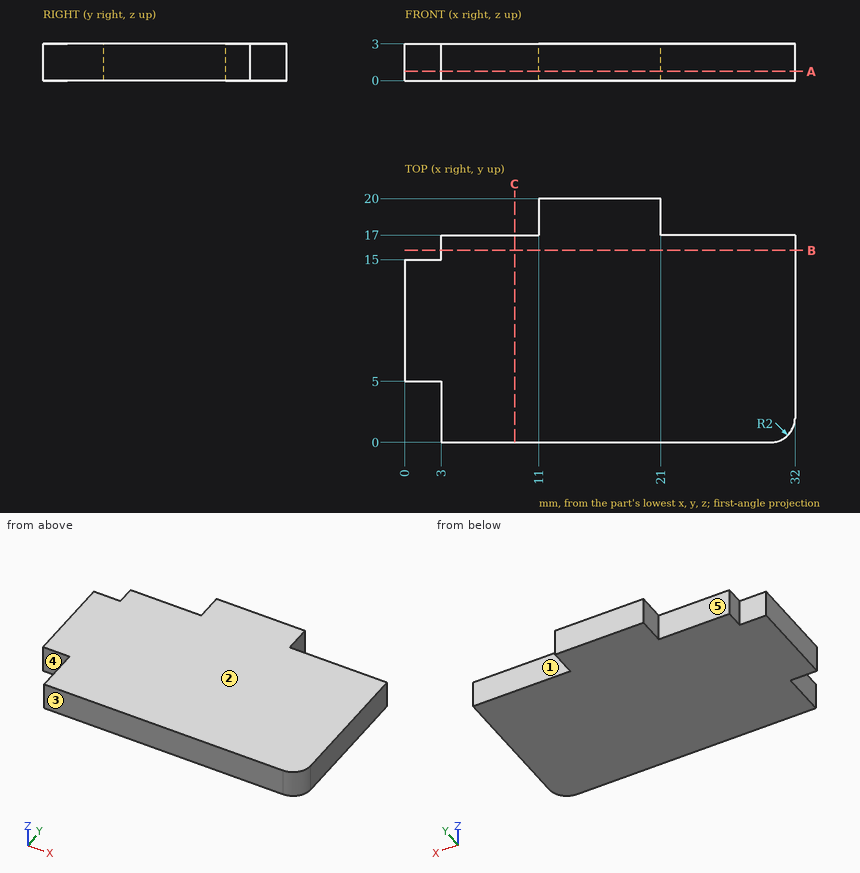
Design review of the part shown in the three views and the two pictorial views. Dimensions are in mm from the part's minimum x, y and z. A direction names the side the tool comes from. Round coordinates to 2 decimals unless told otherwise and drop trailing zeros. Loops run counter-clockwise (first coordinate to the right, second up) from the corner with the lowest first, then second, coordinate; pieces in that order, holes last.
(1) We need section B-B (y = 15.75). Give the boundary of the cut face in (x, z), plus the area to 3 significant figures.
Returned:
outline: (3, 0) - (32, 0) - (32, 3) - (3, 3) - close
area: 87.0 mm2
(2) Tool access review of the marked faces 1, 2, 3, 4 and 5: name each direction out of +Z, -Z, +X, -X, +Y, -Y from which nothing blocks a thin tool from reaching the whole face with its end or side.
Returned:
face 1: +Z, -Z, +X, +Y
face 2: +Z, +X, -X, +Y, -Y
face 3: +Z, -Z, +X, -X, -Y
face 4: +Z, -Z, -X, -Y
face 5: +Z, -Z, -X, +Y
(3) We need section C-C (x = 9). Give the boundary of the cut face in (y, z), plus the area to 3 significant figures.
Returned:
outline: (0, 0) - (17, 0) - (17, 3) - (0, 3) - close
area: 51.0 mm2
(4) We need section A-A (z = 0.75). Give the boundary of the cut face in (x, y), plus the area to 3 significant figures.
Returned:
outline: (0, 5) - (3, 5) - (3, 0) - (30, 0) arc R2 ccw to (32, 2) - (32, 17) - (21, 17) - (21, 20) - (11, 20) - (11, 17) - (3, 17) - (3, 15) - (0, 15) - close
area: 552 mm2
(5) Wall thickness on line 1 along X through (y, z) = (3.75, 0.4); line 2 along Y through (x, z) = (28.5, 0.9); line 3 along X through (y, z) = (18.5, 2.25): over which ranges is each line inside the solid? List them lowest first.
Returned:
line 1: x = 3 to 32
line 2: y = 0 to 17
line 3: x = 11 to 21
(6) Clearance check with flat-ended pins moving along their axes: P1, Ø0.9, axis at x = 2, z = 1.5, coming from the -Y side; P2, Ø1.5, axis at y = 18, z = 1, coming from the +X side; P3, Ø0.9, axis at y = 1.5, z = 2, coming from the -X side. State where each tip first meets the part, or that it passes through.
Returned:
P1: stops at y = 5
P2: stops at x = 21
P3: stops at x = 3
